Verification items for the finished model (mm, model axes). A direction names the side the tool comes from. Coordinates: 2 decimals unless noted, no trailing zeros. Write each loop counter-clockwise with the first axis right and the second up, starting at its lowest first coordinate (ties: lowest second). Pieces come first, ordered by that corner, then holes. Notation, with made-up numbers: (-0.5, 75) -> (38.5, 75) arc R10 ccw to (38.5, 81) -> close; hole circle Ø7 at (11.5, 63.5). An arc over 180 degrees is marked (long way). Answer in a Markdown table with one row per item.
```python
from build123d import *

# Parameters (mm, degrees)
PAD_DEPTH    = 4.6
SKETCH001_W  = 1.6
SKETCH001_H  = 2.5
POCKET_DEPTH = 5.001
CHAMFER_SIZE = 0.5


with BuildPart() as part:
    # Sketch (on XZ_Plane of Origin) → Pad (new body)
    with BuildSketch(Plane.XZ):
        with BuildLine():
            Line((0, 0), (0, 1.75))
            ThreePointArc((5, 1.75), (2.5, 4.25), (0, 1.75))
            Line((5, 1.75), (5, 0))
            Line((5, 0), (0, 0))
        make_face()
    extrude(amount=PAD_DEPTH)

    # Sketch001 (on Face3 of Pad) → Pocket (cut, through all)
    with BuildSketch(Plane.YZ.offset(5)):
        with Locations((-2.3, 3)):
            Rectangle(SKETCH001_W, SKETCH001_H)
    extrude(amount=-POCKET_DEPTH, mode=Mode.SUBTRACT)

    # Chamfer
    chamfer_edges = [part.edges().sort_by_distance(p)[0] for p in [
        (2.5, -4.6, 4.25),
        (2.5, -4.6, 0),
        (2.5, 0, 4.25),
        (5, -2.3, 0),
        (2.5, 0, 0),
        (0, -2.3, 0),
    ]]
    chamfer(chamfer_edges, length=CHAMFER_SIZE)


solid = part.part
```
1. Section check B-B, the plane y = -2.9. Record the boundary of the cut face in (x, z), plus the area to 3 significant figures.
Geometry says:
| item | result |
|---|---|
| outline | (0, 0.5) -> (0.5, 0) -> (4.5, 0) -> (5, 0.5) -> (5, 1.75) -> (0, 1.75) -> close |
| area | 8.50 mm^2 |
2. Section check C-C, the plane z = 1.4. Record the boundary of the cut face in (x, y), plus the area to 3 significant figures.
Geometry says:
| item | result |
|---|---|
| outline | (0, -4.1) -> (0.5, -4.6) -> (4.5, -4.6) -> (5, -4.1) -> (5, -0.5) -> (4.5, 0) -> (0.5, 0) -> (0, -0.5) -> close |
| area | 22.5 mm^2 |
3. Section check D-D, the plane y = -3.8. Record the boundary of the cut face in (x, z), plus the area to 3 significant figures.
Geometry says:
| item | result |
|---|---|
| outline | (0, 0.5) -> (0.5, 0) -> (4.5, 0) -> (5, 0.5) -> (5, 1.75) arc R2.5 ccw to (0, 1.75) -> close |
| area | 18.3 mm^2 |
4. Mould release check, pull along Y, two halves, no side actions. Record for faces 1 (the flat face through (3, -4.6, 2)), 2 (the flat face through (3, -1.5, 3)), 3 (the cylindrical face through (2.55, -3.59, 4.25)), 4 (the flat face through (3, 0, 2)): released by +Y, released by -Y, zero draft, split by the parting line, or undercut.
Geometry says:
| item | result |
|---|---|
| face 1 | released by -Y |
| face 2 | undercut |
| face 3 | zero draft |
| face 4 | released by +Y |
5. Section check A-A, the plane x = 2.5. Record the boundary of the cut face in (y, z), plus the area to 4 significant figures.
Geometry says:
| item | result |
|---|---|
| outline | (-4.6, 0.5) -> (-4.1, 0) -> (-0.5, 0) -> (0, 0.5) -> (0, 3.75) -> (-0.5, 4.25) -> (-1.5, 4.25) -> (-1.5, 1.75) -> (-3.1, 1.75) -> (-3.1, 4.25) -> (-4.1, 4.25) -> (-4.6, 3.75) -> close |
| area | 15.05 mm^2 |
6. Tool access check on faces 5 (the flat face through (5, -2, 1)), 6 (the flat face through (3, -2, 1.75)). Record the directions out of +Z, -Z, +X, -X, +Y, -Y that give a thin tool (end or side, any length) a straight path to the whole face; none if there is none.
Geometry says:
| item | result |
|---|---|
| face 5 | +Z, -Z, +X, +Y, -Y |
| face 6 | +Z, +X, -X |
7. Depth check by flat-ended pin: P1, Ø0.8, axis at x = 1.5, y = -2, coming from the +Z side. Enter the tip coordinate at first touch or a pass-through.
Geometry says:
| item | result |
|---|---|
| P1 | z = 1.75 |
8. Thickness scan on line 1 (Y direction, x = 3.1, z = 2.8); line 2 (Y direction, x = 0.5, z = 2.5); line 3 (Z direction, x = 0.8, y = -2.7). Record the ranges inside material, lowest first. Write a range as from..to.
Geometry says:
| item | result |
|---|---|
| line 1 | -4.6..-3.1, -1.5..0 |
| line 2 | -4.46..-3.1, -1.5..-0.14 |
| line 3 | 0..1.75 |
